from build123d import *

# Parameters (mm, degrees)
SKETCH_1_W          = 720
SKETCH_1_H          = 520
EXTRUDE_1_DEPTH     = 5
CUT_EXTRUDE_1_DEPTH = 445.100213916
SKETCH_3_R          = 2.5
CUT_EXTRUDE_2_DEPTH = 445.100213916
SKETCH_4_W          = 20
SKETCH_4_H          = 20
CUT_EXTRUDE_3_DEPTH = 10
FILLET_1_R          = 5


with BuildPart() as part:
    # 草图1 → 凸台-拉伸1 (new body)
    with BuildSketch(Plane.XY):
        Rectangle(SKETCH_1_W, SKETCH_1_H)
    extrude(amount=EXTRUDE_1_DEPTH)

    # 草图2 → 切除-拉伸1 (cut, through all)
    with BuildSketch(Plane.XY.offset(5)):
        Polygon((340, -240), (340, -200), (360, -200), (360, -260), (300, -260), (300, -240), align=None)
        Polygon((340, 240), (300, 240), (300, 260), (360, 260), (360, 200), (340, 200), align=None)
        Polygon((-340, 240), (-340, 200), (-360, 200), (-360, 260), (-300, 260), (-300, 240), align=None)
        Polygon((-340, -240), (-300, -240), (-300, -260), (-360, -260), (-360, -200), (-340, -200), align=None)
    extrude(amount=-CUT_EXTRUDE_1_DEPTH, mode=Mode.SUBTRACT)

    # 草图3 → 切除-拉伸2 (cut, through all)
    with BuildSketch(Plane.XY.offset(5)):
        with Locations((350, 180)):
            Circle(SKETCH_3_R)
        with Locations((280, 250)):
            Circle(SKETCH_3_R)
        with Locations((-280, 250)):
            Circle(SKETCH_3_R)
        with Locations((-350, 180)):
            Circle(SKETCH_3_R)
        with Locations((-350, -180)):
            Circle(SKETCH_3_R)
        with Locations((-280, -250)):
            Circle(SKETCH_3_R)
        with Locations((350, -180)):
            Circle(SKETCH_3_R)
        with Locations((280, -250)):
            Circle(SKETCH_3_R)
    extrude(amount=-CUT_EXTRUDE_2_DEPTH, mode=Mode.SUBTRACT)

    # 草图4 → 切除-拉伸3 (cut)
    with BuildSketch(Plane.XY.offset(5)):
        with Locations((23, 250)):
            Rectangle(SKETCH_4_W, SKETCH_4_H)
    cut_extrude_3 = extrude(amount=-CUT_EXTRUDE_3_DEPTH, mode=Mode.SUBTRACT)

    # 镜向2: 切除-拉伸3 across plane
    add(cut_extrude_3.mirror(Plane.ZX), mode=Mode.SUBTRACT)

    # 圆角1
    fillet_1_edges = [part.edges().sort_by_distance(p)[0] for p in [
        (13, 260, 2.5),
        (33, 260, 2.5),
        (33, 240, 2.5),
        (13, 240, 2.5),
        (33, -260, 2.5),
        (13, -260, 2.5),
        (13, -240, 2.5),
        (33, -240, 2.5),
        (-360, -200, 2.5),
        (-340, -200, 2.5),
        (-340, -240, 2.5),
        (-300, -240, 2.5),
        (-300, -260, 2.5),
        (-300, 260, 2.5),
        (-300, 240, 2.5),
        (-340, 240, 2.5),
        (-340, 200, 2.5),
        (-360, 200, 2.5),
        (360, 200, 2.5),
        (340, 200, 2.5),
        (340, 240, 2.5),
        (300, 240, 2.5),
        (300, 260, 2.5),
        (300, -260, 2.5),
        (300, -240, 2.5),
        (340, -240, 2.5),
        (340, -200, 2.5),
        (360, -200, 2.5),
    ]]
    fillet(fillet_1_edges, radius=FILLET_1_R)


solid = part.part
The listing builds one solid part. Answer for the finished solid, in the listing's coordinates (mm). Coordinates: 2 decimals unless noted, no trailing zeros. Answer in a Markdown table with one row per item.
1) Find the intervals of material crossed by probe 1 along Y at (x, z) = (280, 1.15); probe 2 along X at (y, z) = (250, 1.2); probe 3 along X at (y, z) = (-180, 1.9), in increasing order.
Answers below:
| item | result |
|---|---|
| probe 1 | -260 to -252.5, -247.5 to 247.5, 252.5 to 260 |
| probe 2 | -300 to -282.5, -277.5 to 13, 33 to 277.5, 282.5 to 300 |
| probe 3 | -360 to -352.5, -347.5 to 347.5, 352.5 to 360 |
2) Find section A-A (z = 2.95). Count the separate pieces of the cut face and the enclosed holes in it, then the cut area to 3 significant figures.
Answers below:
| item | result |
|---|---|
| separate pieces | 1 |
| enclosed holes | 8 |
| area | 365,000 mm^2 |
3) Given pin 1 (2.5 mm diameter, centred on y = 250.5, z = 3, fed in from -X); pin 2 (6 mm diameter, centred on x = -280, y = 250, fed in from +Z); pin 3 (1.5 mm diameter, centred on x = -351, z = 1.5, fed in from -Y); pin 4 (1.5 mm diameter, centred on y = 217, z = 1.5, fed in from +X), each flat-ended and moving along its own axis, determine where each tip first touches the part or whether it passes through.
Answers below:
| item | result |
|---|---|
| pin 1 | x = -300 |
| pin 2 | z = 5 |
| pin 3 | y = -200 |
| pin 4 | x = 340 |
